Read the model definition and answer for the solid it produces. Units are mm, in the model's axes. A direction names the side the tool comes from. Coordinates: 2 decimals unless noted, no trailing zeros. Write each loop counter-clockwise with the first axis right and the second up, starting at its lowest first coordinate (ties: lowest second). Pieces come first, ordered by that corner, then holes. Notation, with made-up numbers: (19.25, 22.25) -> (51.25, 22.25) arc R14 cw to (51.25, 28.25) -> close; hole circle Ø11 at (-3, -8.5). An arc over 180 degrees is marked (long way). Answer in a Markdown table with one row per item. Add a question column.
Item 1: For a pull along X with two mould halves and no side action, classify faces 4 (the face through (0, -13, 9.5)), 5 (the face through (0, -14, -7.9)), 6 (the face through (-9.5, -17, 0)), 7 (the face through (0, -14, 7.9)) as +X half, -X half, draft (parallel to the pull), parting line (faces both ways), or undercut.
Item 2: Straight lines are drawn through the part: line 1 (Y direction, x = -4.25, z = -6); line 2 (Y direction, x = -7.25, z = -8.75); line 3 (X direction, y = -16.5, z = -5.5). For each, find the intervals that lie inside material, in ascending order. Write a range as from..to.
Item 3: Which of the six approach directions +Z, -Z, +X, -X, +Y, -Y give full straight-line access (tool end or side, diameter ignored) to faces 1 (the face through (0.175, -9.793, 0.359)), 2 (the face through (0.175, 8.999, -5.196)), 3 (the face through (7.9, -17, 0))?
Item 4: Section D-D on z = 8.5 is taken. Write down the section's boundary in (x, y), then the cut area to 3 significant figures.
Item 5: Section B-B on y = 0 is taken. Write down the section's boundary in (x, z).
Item 6: Given pin 1 Ø2 at (y, z) = (-17, -3) entering from -X; pin 2 Ø8 at (y, z) = (-19, 0) entering from +X; pin 3 Ø5 at (x, y) = (6.5, -1) entering from -Z, each flat-ended and moving along its own axis, determine where each tip first touches the part or whether it passes through.
Item 7: Section A-A on x = 0 is taken. Write down the section's boundary in (y, z), then the cut area to 3 significant figures.
Item 8: Section C-C on z = 0 is taken. Write down the section's boundary in (x, y), then the cut area to 3 significant figures.
```python
from build123d import *

# Parameters (mm, degrees)
BOSS_EXTRUDE1_DEPTH = 12.5
SKETCH3_W           = 19
SKETCH3_H           = 19
SKETCH3_W_2         = 15.8
SKETCH3_H_2         = 15.8
BOSS_EXTRUDE3_DEPTH = 25
SKETCH2_R           = 11
SKETCH2_R_2         = 9.4
BOSS_EXTRUDE2_DEPTH = 12.5
SKETCH4_R           = 9.8
CUT_EXTRUDE1_DEPTH  = 20
SKETCH5_R           = 9.4
CUT_EXTRUDE2_DEPTH  = 20


with BuildPart() as part:
    # Sketch1 → Boss-Extrude1 (new, symmetric)
    with BuildSketch(Plane(origin=(0, 0, 0), x_dir=(0, 0, -1), z_dir=(1, 0, 0))):
        with BuildLine():
            Line((-5.5, 9.526279442), (-4.9, 8.487048957))
            ThreePointArc((-4.9, 8.487048957), (0, -9.8), (4.9, 8.487048957))
            Line((4.9, 8.487048957), (5.5, 9.526279442))
            ThreePointArc((5.5, 9.526279442), (0, -11), (-5.5, 9.526279442))
        make_face()
    extrude(amount=BOSS_EXTRUDE1_DEPTH, both=True)

    # Sketch3 → Boss-Extrude3 (add)
    with BuildSketch(Plane(origin=(0, 0, 0), x_dir=(1, 0, 0), z_dir=(0, 1, 0))):
        Rectangle(SKETCH3_W, SKETCH3_H)
        Rectangle(SKETCH3_W_2, SKETCH3_H_2, mode=Mode.SUBTRACT)
    extrude(amount=-BOSS_EXTRUDE3_DEPTH)

    # Sketch2 → Boss-Extrude2 (add, symmetric)
    with BuildSketch(Plane.XY):
        with Locations((0, -31)):
            Circle(SKETCH2_R)
        with Locations((0, -31)):
            Circle(SKETCH2_R_2, mode=Mode.SUBTRACT)
    extrude(amount=BOSS_EXTRUDE2_DEPTH, both=True)

    # Sketch4 → Cut-Extrude1 (cut, symmetric)
    with BuildSketch(Plane(origin=(0, 0, 0), x_dir=(0, 0, -1), z_dir=(1, 0, 0))):
        Circle(SKETCH4_R)
    extrude(amount=CUT_EXTRUDE1_DEPTH, both=True, mode=Mode.SUBTRACT)

    # Sketch5 → Cut-Extrude2 (cut, symmetric)
    with BuildSketch(Plane.XY):
        with Locations((0, -31)):
            Circle(SKETCH5_R)
    extrude(amount=CUT_EXTRUDE2_DEPTH, both=True, mode=Mode.SUBTRACT)


solid = part.part
```
Results below:
| question | item | result |
|---|---|---|
| 1 | face 4 | draft |
| 1 | face 5 | undercut |
| 1 | face 6 | -X half |
| 1 | face 7 | undercut |
| 2 | line 1 | y = -41.15..-39.38, -22.62..-20.85, -9.22..-7.75, 7.75..9.22 |
| 2 | line 2 | y = -39.27..-36.98, -25.02..-4.41, 4.41..6.67 |
| 2 | line 3 | x = -9.5..-7.9, 7.9..9.5 |
| 3 | face 1 | +X, -X |
| 3 | face 2 | +X, -X, +Y |
| 3 | face 3 | none |
| 4 | outline | (-12.5, -6.98) -> (-9.5, -6.98) -> (-9.5, -25) -> (-9.22, -25) arc R11 ccw (long way) to (9.22, -25) -> (9.5, -25) -> (9.5, -6.98) -> (12.5, -6.98) -> (12.5, -4.88) -> (-12.5, -4.88) -> close; (-12.5, 4.88) -> (12.5, 4.88) -> (12.5, 6.98) -> (-12.5, 6.98) -> close; hole circle Ø18.8 at (0, -31) |
| 4 | area | 485 mm2 |
| 5 | outline | (-12.5, -11) -> (12.5, -11) -> (12.5, -9.8) -> (-12.5, -9.8) -> close; (-12.5, 9.8) -> (12.5, 9.8) -> (12.5, 11) -> (-12.5, 11) -> close |
| 6 | pin 1 | stops at x = -9.5 |
| 6 | pin 2 | stops at x = 9.5 |
| 6 | pin 3 | stops at z = -11 |
| 7 | outline | (-42, -12.5) -> (-40.4, -12.5) -> (-40.4, 12.5) -> (-42, 12.5) -> close; (-21.6, -12.5) -> (-20, -12.5) -> (-20, -9.5) -> (-5.55, -9.5) arc R11 ccw to (9.53, -5.5) -> (8.49, -4.9) arc R9.8 cw (long way) to (8.49, 4.9) -> (9.53, 5.5) arc R11 ccw to (-5.55, 9.5) -> (-20, 9.5) -> (-20, 12.5) -> (-21.6, 12.5) -> close; hole (-20, -7.9) -> (-7.65, -7.9) arc R11 cw to (-7.65, 7.9) -> (-20, 7.9) -> close |
| 7 | area | 188 mm2 |
| 8 | outline | (-12.5, -11) -> (-9.5, -11) -> (-9.5, -25) -> (-9.22, -25) arc R11 ccw (long way) to (9.22, -25) -> (9.5, -25) -> (9.5, -11) -> (12.5, -11) -> (12.5, -9.8) -> (-12.5, -9.8) -> close; hole circle Ø18.8 at (0, -31); hole (-7.9, -23.35) arc R11 cw to (7.9, -23.35) -> (7.9, -11) -> (-7.9, -11) -> close |
| 8 | area | 175 mm2 |
